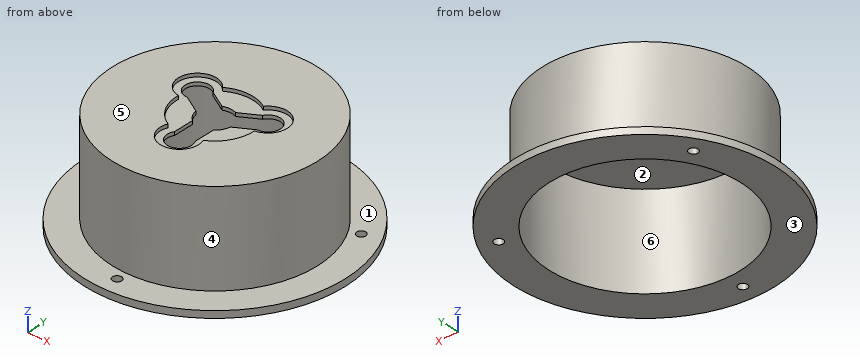
Solid Edge part; units mm, degrees
sketch "Sketch1" plane through (0, 0, 0) normal (0, 0, 1) x (1, 0, 0)
  circle A0 centre (0, 0) radius 37.5
  circle A1 centre (0, 0) radius 27.5
extrude "Protrusion1" add sketch "Sketch1" along normal blind 2
sketch "Sketch2" plane through (0, 0, 2) normal (0, 0, 1) x (1, 0, 0)
  circle A0 centre (0, 0) radius 27.5
  circle A1 centre (0, 0) radius 29.5
extrude "Cup" add sketch "Sketch2" along normal blind 27
sketch "Sketch3" plane through (0, 0, 29) normal (0, 0, 1) x (1, 0, 0)
  circle A0 centre (0, 0) radius 27.5
extrude "End" add sketch "Sketch3" against normal blind 2
hole "Attachment___Edge" at (0, -32.5, 0) direction (0, 0, 1) diameter 2.6 end up to next
pattern_circular "Pattern1" count 3 over 360 about axis through (0, 0, 0) along (0, 0, 1) of "Attachment___Edge"
sketch "Sketch4" plane through (0, 0, 29) normal (0, 0, 1) x (-1, 0, 0)
  line L0 (-10.1603, -2.4019) -> (-4.9641, 0.5981)
  line L1 (-3, 4) -> (-3, 10)
  line L2 (3, 10) -> (3, 4)
  arc A0 (3, 4) -> (4.9641, 0.5981) centre (0, 0) cw
  line L3 (4.9641, 0.5981) -> (10.1603, -2.4019)
  line L4 (7.1603, -7.5981) -> (1.9641, -4.5981)
  arc A1 (1.9641, -4.5981) -> (-1.9641, -4.5981) centre (0, 0) cw
  line L5 (-7.1603, -7.5981) -> (-1.9641, -4.5981)
  arc A2 (10.1603, -2.4019) -> (7.1603, -7.5981) centre (10.2215, -5.9014) cw
  arc A3 (-3, 10) -> (3, 10) centre (0, 11.8028) cw
  arc A4 (-4.9641, 0.5981) -> (-3, 4) centre (0, 0) cw
  arc A5 (-7.1603, -7.5981) -> (-10.1603, -2.4019) centre (-10.2215, -5.9014) cw
  dimension "D1" = 10.1603
extrude "Cutout1" cut sketch "Sketch4" against normal up to next
sketch "Sketch5" plane through (0, 0, 29) normal (0, 0, 1) x (-1, 0, 0)
  arc A0 (-5.1009, 9.7458) -> (5.1009, 9.7458) centre (0, 11.8028) cw
  arc A1 (5.1009, 9.7458) -> (10.9906, -0.4554) centre (0, 0) cw
  arc A2 (10.9906, -0.4554) -> (5.8897, -9.2904) centre (10.2215, -5.9014) cw
  arc A3 (-5.8897, -9.2904) -> (-10.9906, -0.4554) centre (-10.2215, -5.9014) cw
  arc A4 (-10.9906, -0.4554) -> (-5.1009, 9.7458) centre (0, 0) cw
  arc A5 (5.8897, -9.2904) -> (-5.8897, -9.2904) centre (0, 0) cw
extrude "Cutout_distance___End" cut sketch "Sketch5" against normal blind 1
properties material "ABS Plastic, medium impact"
Model file for the job. Use its own axes, mm. Face numbers are marked on the shaded views. A direction names the side the tool comes from. Round coordinates to 2 decimals unless told otherwise and drop trailing zeros. Loops run counter-clockwise (first coordinate to the right, second up) from the corner with the lowest first, then second, coordinate; pieces in that order, holes last. Notation, with made-up numbers: (3.25, 25) - (26.25, 25) arc R20 ccw to (26.25, 33) - close; hole circle Ø4 at (42, 34). An arc over 180 degrees is marked (long way). Write each question's results on one line, items separated by ' | '.
(1) Saw through at B-B, the plane y = -32.5. List the corners of the cut face in (x, z), then the cut area to 3 significant figures.
Answer below:
outline: (-18.71, 0) - (-1.3, 0) - (-1.3, 2) - (-18.71, 2) - close; (1.3, 0) - (18.71, 0) - (18.71, 2) - (1.3, 2) - close | area: 69.6 mm^2
(2) Saw through at A-A, the plane x = 0. List the corners of the cut face in (y, z), then the cut area to 3 significant figures.
Answer below:
outline: (-37.5, 0) - (-33.8, 0) - (-33.8, 2) - (-37.5, 2) - close; (-31.2, 0) - (-27.5, 0) - (-27.5, 27) - (-15.3, 27) - (-15.3, 28) - (-17.3, 28) - (-17.3, 29) - (-29.5, 29) - (-29.5, 2) - (-31.2, 2) - close; (5, 27) - (27.5, 27) - (27.5, 0) - (37.5, 0) - (37.5, 2) - (29.5, 2) - (29.5, 29) - (11, 29) - (11, 28) - (5, 28) - close | area: 204 mm^2
(3) Saw through at D-D, the plane z = 8.75. List the corners of the cut face in (x, y).
Answer below:
outline: circle Ø59 at (0, 0); hole circle Ø55 at (0, 0)
(4) Saw through at C-C, the plane x = -8.5. List the corners of the cut face in (y, z).
Answer below:
outline: (-36.52, 0) - (-26.15, 0) - (-26.15, 27) - (1.44, 27) - (1.44, 28) - (-6.98, 28) - (-6.98, 29) - (-28.25, 29) - (-28.25, 2) - (-36.52, 2) - close; (8.95, 27) - (26.15, 27) - (26.15, 0) - (36.52, 0) - (36.52, 2) - (28.25, 2) - (28.25, 29) - (11.13, 29) - (11.13, 28) - (8.95, 28) - close
(5) Wall check: L1, parallel to X at y = 16.25, z = 1; L2, parallel to Y at x = 0, z = 28.55; L3, parallel to Z at x = 2, y = -26. Give the ranges that are in metal, low to high.
Answer below:
L1: x = -33.8 to -29.45, -26.85 to -22.19, 22.19 to 26.85, 29.45 to 33.8 | L2: y = -29.5 to -17.3, 11 to 29.5 | L3: z = 27 to 29
(6) 3-axis set-ups, long thin cutter, end or side, ignore diameter. For the marked faces 1, 2 and 3: which of +Z, -Z, +X, -X, +Y, -Y reach the whole face in a straight line?
Answer below:
face 1: +Z | face 2: -Z | face 3: -Z, +X, -X, +Y, -Y
(7) Mould opens along Y. For the marked faces 4, 5 and 6 say: released by +Y, released by -Y, zero draft, split by the parting line, or undercut.
Answer below:
face 4: split by the parting line | face 5: zero draft | face 6: undercut
(8) Pin check, flat tips, straight feed: pin 1 (3 mm diameter, centred on x = 8, z = 16, fed in from +Y) (3 decimals); pin 2 (12.5 mm diameter, centred on x = -10.22, y = 5.9, fed in from -Z); pin 3 (4 mm diameter, centred on y = 19, z = 11, fed in from -X). Stop position of each tip, or through.
Answer below:
pin 1: stops at y = 28.775 | pin 2: stops at z = 27 | pin 3: stops at x = -24.11
